Read the model definition and answer for the solid it produces. Units are mm, in the model's axes. Round coordinates to 2 decimals unless told otherwise and drop trailing zeros. Write each loop counter-clockwise with the first axis right and the second up, starting at its lowest first coordinate (ties: lowest second). Pieces come first, ordered by that corner, then holes. Notation, with made-up numbers: (21, 65.5) - (62, 65.5) arc R20 cw to (62, 101.5) - close; hole circle Ø9 at (4, 27). An arc over 180 degrees is marked (long way). One line per item, written item: value. Start each with the question number.
(1) A cutting plane is placed at A-A, the plane z = 30.48. Determine the outline of the cut face in (x, y) (3 decimals), plus the area to 3 significant figures.
(2) A cutting plane is placed at C-C, the plane x = 0. Determine the outline of the cut face in (y, z) (3 decimals).
(3) Flat-ended cylindrical pins translate along their axes: pin 1 Ø3.5 at (x, z) = (30.48, 30.48) entering from +Y; pin 2 Ø5.5 at (x, z) = (-30.48, 30.48) entering from +Y. Find the tip coordinate at first contact, or state that the pin passes through.
(4) Find the intervals of material crossed by L1, parallel to Z at x = 30.48, y = 0.7; L2, parallel to X at y = 0.5, z = 31; L3, parallel to X at y = 2.2, z = 23, in increasing order.
(5) A cutting plane is placed at D-D, the plane y = 0.75. State how many separate pieces and enclosed holes the cut face has, plus the area to 3 significant figures.
(6) A cutting plane is placed at B-B, the plane x = 30.48. Determine the outline of the cut face in (y, z) (3 decimals), plus the area to 3 significant figures.
from build123d import *

# Parameters (mm, degrees)
SKETCH1_W                        = 73.66
SKETCH1_H                        = 73.66
SKETCH1_R                        = 3.175
BOSS_EXTRUDE1_DEPTH              = 3.175
CHAMFER2_SIZE                    = 2.54
F_10_32_TAPPED_HOLE1_D           = 4.0386
F_10_32_TAPPED_HOLE1_CSINK_D     = 6.096
F_10_32_TAPPED_HOLE1_CSINK_ANGLE = 90
F_10_32_TAPPED_HOLE2_D           = 4.0386
F_10_32_TAPPED_HOLE2_CSINK_D     = 6.096
F_10_32_TAPPED_HOLE2_CSINK_ANGLE = 90


with BuildPart() as part:
    # Sketch1 → Boss-Extrude1 (new body)
    with BuildSketch(Plane(origin=(0, 0, 0), x_dir=(1, 0, 0), z_dir=(0, 1, 0))):
        Rectangle(SKETCH1_W, SKETCH1_H)
        with Locations(Location((0, 0, 0), (0, 0, 270))):
            Circle(SKETCH1_R, mode=Mode.SUBTRACT)
    extrude(amount=BOSS_EXTRUDE1_DEPTH)

    # Chamfer2
    chamfer2_edges = [part.edges().sort_by_distance(p)[0] for p in [
        (-36.83, 1.5875, -36.83),
        (36.83, 1.5875, -36.83),
        (36.83, 1.5875, 36.83),
        (-36.83, 1.5875, 36.83),
    ]]
    chamfer(chamfer2_edges, length=CHAMFER2_SIZE)

    # #10-32 Tapped Hole1 (through all)
    with Locations(Plane(origin=(0, 3.175, 0), x_dir=(1, 0, 0), z_dir=(0, 1, 0))):
        with Locations((30.48, 30.48), (-30.48, 30.48), (-30.48, -30.48), (30.48, -30.48)):
            CounterSinkHole(F_10_32_TAPPED_HOLE1_D / 2, F_10_32_TAPPED_HOLE1_CSINK_D / 2, counter_sink_angle=F_10_32_TAPPED_HOLE1_CSINK_ANGLE)

    # #10-32 Tapped Hole2 (through all)
    with Locations(Plane(origin=(0, 3.175, 0), x_dir=(1, 0, 0), z_dir=(0, 1, 0))):
        with Locations((-24.765, 24.765), (24.765, 24.765), (-24.765, -24.765), (24.765, -24.765)):
            CounterSinkHole(F_10_32_TAPPED_HOLE2_D / 2, F_10_32_TAPPED_HOLE2_CSINK_D / 2, counter_sink_angle=F_10_32_TAPPED_HOLE2_CSINK_ANGLE)


solid = part.part
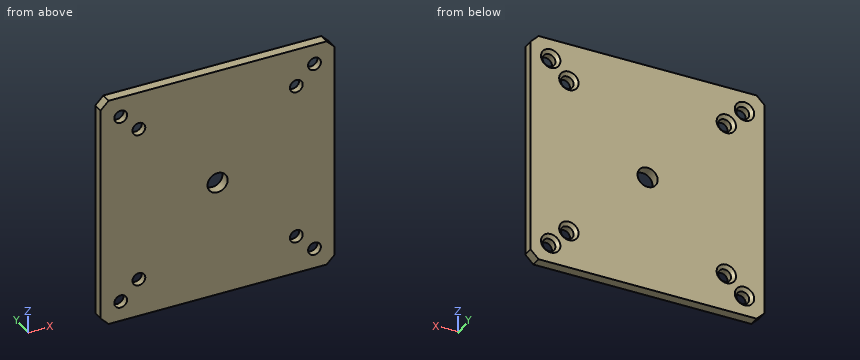
Here are the results:
1. outline: (-36.83, 0) - (-32.499, 0) - (-32.499, 2.146) - (-33.528, 3.175) - (-36.83, 3.175) - close; (-28.461, 0) - (28.461, 0) - (28.461, 2.146) - (27.432, 3.175) - (-27.432, 3.175) - (-28.461, 2.146) - close; (32.499, 0) - (36.83, 0) - (36.83, 3.175) - (33.528, 3.175) - (32.499, 2.146) - close
1. area: 206 mm²
2. outline: (0, -36.83) - (3.175, -36.83) - (3.175, -3.175) - (0, -3.175) - close; (0, 3.175) - (3.175, 3.175) - (3.175, 36.83) - (0, 36.83) - close
3. pin 1: through
3. pin 2: y = 2.88
4. L1: -36.83 to -32.5, -28.46 to 28.46, 32.5 to 36.83
4. L2: -36.83 to -32.43, -28.53 to 28.53, 32.43 to 36.83
4. L3: -36.83 to -25.85, -23.68 to 23.68, 25.85 to 36.83
5. separate pieces: 1
5. enclosed holes: 9
5. area: 5,280 mm²
6. outline: (0, -36.83) - (3.175, -36.83) - (3.175, -33.528) - (2.146, -32.499) - (0, -32.499) - close; (0, -28.461) - (2.146, -28.461) - (3.175, -27.432) - (3.175, 27.432) - (2.146, 28.461) - (0, 28.461) - close; (0, 32.499) - (2.146, 32.499) - (3.175, 33.528) - (3.175, 36.83) - (0, 36.83) - close
6. area: 206 mm²
